Here's how the part is built. I have some questions about the finished solid (model axes, mm). Face numbers are marked on the shaded views. A direction names the side the tool comes from. Coordinates: 2 decimals unless noted, no trailing zeros. Write each loop counter-clockwise with the first axis right and the second up, starting at its lowest first coordinate (ties: lowest second). Pieces come first, ordered by that corner, then holes. Notation, with made-up numbers: M 21.5,-30 L 39.5,-30 A20 ccw 39.5,-10 Z; hole C 28,86.5 d3. An arc over 180 degrees is marked long. Use one line per item in the form item = value. Start each with the question number.
1. I want a section at D-D, the plane y = 8.5. List the corners of the cut face in (x, z) for me, plus the area to 3 significant figures.
2. I want a section at B-B, the plane z = 0. List the corners of the cut face in (x, y) for me.
3. Thinking about a two-plate mould opening in X: for the marked faces 1, 2 and 3, which applies, released by +X, released by -X, zero draft, split by the parting line, or undercut?
4. I'm going to push a flat-ended pin straight in: pin 1 Ø3 at (y, z) = (6, -3) entering from +X. Where does the tip first touch, or does it pass through?
5. On a 3-axis mill with a long thin cutter (end or side, diameter ignored), from which of +Z, -Z, +X, -X, +Y, -Y can I reach the whole of each face in a straight line? I mean the marked faces 4 and 5. Say none if no direction works.
6. I want a section at C-C, the plane x = 3. List the corners of the cut face in (y, z) for me, plus the area to 3 significant figures.
7. I want a section at A-A, the plane x = 0. List the corners of the cut face in (y, z) for me, plus the area to 3 significant figures.
8. Please list where these lines run through material, in increasing order: line 1 along Z through (x, y) = (0, 5.75); line 2 along Y through (x, z) = (0.5, -3.75); line 3 along Z through (x, y) = (0.75, 1.5). Write a range as [from, to].
from build123d import *

# Parameters (mm, degrees)
SKETCH1_R                  = 3.75
BOSS_EXTRUDE1_DEPTH        = 10.5
F_3_5_3_5_DIAMETER_HOLE1_D = 3.5
SKETCH5_R                  = 4.75
SKETCH5_R_2                = 3.75
BOSS_EXTRUDE2_DEPTH        = 2.5


with BuildPart() as part:
    # Sketch1 → Boss-Extrude1 (new body)
    with BuildSketch(Plane(origin=(0, 0, 0), x_dir=(1, 0, 0), z_dir=(0, 1, 0))):
        Circle(SKETCH1_R)
    extrude(amount=BOSS_EXTRUDE1_DEPTH)

    # Ø3.5 (3.5) Diameter Hole1 (through all)
    with Locations(Plane(origin=(0, 10.5, 0), x_dir=(1, 0, 0), z_dir=(0, 1, 0))):
        with Locations((0, 0)):
            Hole(F_3_5_3_5_DIAMETER_HOLE1_D / 2)

    # Sketch5 → Boss-Extrude2 (add)
    with BuildSketch(Plane.XZ):
        Circle(SKETCH5_R)
        Circle(SKETCH5_R_2, mode=Mode.SUBTRACT)
    extrude(amount=-BOSS_EXTRUDE2_DEPTH)


solid = part.part
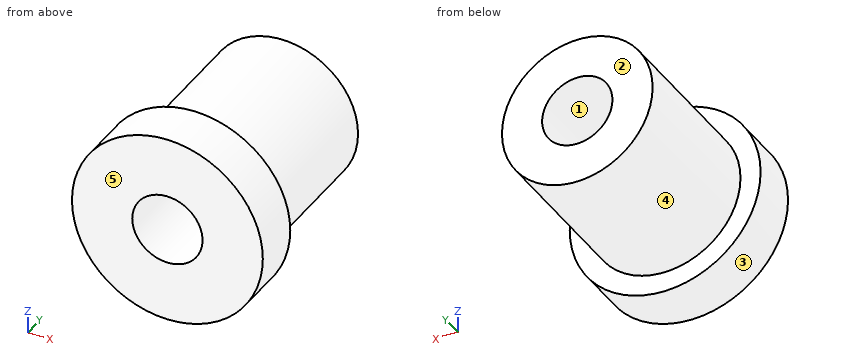
Answer list:
q1.outline = C 0,0 d7.5; hole C 0,0 d3.5
q1.area = 34.6 mm²
q2.outline = M -4.75,0 L -1.75,0 L -1.75,10.5 L -3.75,10.5 L -3.75,2.5 L -4.75,2.5 Z; M 1.75,0 L 4.75,0 L 4.75,2.5 L 3.75,2.5 L 3.75,10.5 L 1.75,10.5 Z
q3.face_1 = undercut
q3.face_2 = zero draft
q3.face_3 = split by the parting line
q4.pin_1 = 3.44
q5.face_4 = +Y
q5.face_5 = +Z, -Z, +X, -X, -Y
q6.outline = M 0,-3.68 L 2.5,-3.68 L 2.5,-2.25 L 10.5,-2.25 L 10.5,2.25 L 2.5,2.25 L 2.5,3.68 L 0,3.68 Z
q6.area = 54.4 mm²
q7.outline = M 0,-4.75 L 2.5,-4.75 L 2.5,-3.75 L 10.5,-3.75 L 10.5,-1.75 L 0,-1.75 Z; M 0,1.75 L 10.5,1.75 L 10.5,3.75 L 2.5,3.75 L 2.5,4.75 L 0,4.75 Z
q7.area = 47.0 mm²
q8.line_1 = [-3.75, -1.75], [1.75, 3.75]
q8.line_2 = [0, 2.5]
q8.line_3 = [-4.69, -1.58], [1.58, 4.69]
